Autodesk Inventor part; units mm, degrees
ref_plane "YZ Plane" through (0, 0, 0) normal (1, 0, 0) x (0, 1, 0)
ref_plane "XZ Plane" through (0, 0, 0) normal (0, 1, 0) x (-1, 0, 0)
ref_plane "XY Plane" through (0, 0, 0) normal (0, 0, 1) x (1, 0, 0)
ref_plane "Work Plane1" through (0, 0, 0) normal (0, 0, 1) x (1, 0, 0)
sketch "Sketch1" plane through (0, 0, 0) normal (0, 0, 1) x (1, 0, 0)
  circle A0 centre (11.5562, -18) radius 2 construction
  line L0 (-53.1938, -16) -> (-53.1938, -30) construction
  arc A1 (-56.1938, -30) -> (-53.1938, -30) centre (-54.6938, -30) ccw construction
  line L1 (-56.1938, -30) -> (-56.1938, -16) construction
  arc A2 (-53.1938, -16) -> (-56.1938, -16) centre (-54.6938, -16) ccw construction
  line L2 (7.0562, -16) -> (7.0562, -30) construction
  arc A3 (4.0562, -30) -> (7.0562, -30) centre (5.5562, -30) ccw construction
  line L3 (4.0562, -30) -> (4.0562, -16) construction
  arc A4 (7.0562, -16) -> (4.0562, -16) centre (5.5562, -16) ccw construction
  line L4 (-13.1938, -16) -> (-13.1938, -30) construction
  arc A5 (-16.1938, -30) -> (-13.1938, -30) centre (-14.6938, -30) ccw construction
  line L5 (-16.1938, -30) -> (-16.1938, -16) construction
  arc A6 (-13.1938, -16) -> (-16.1938, -16) centre (-14.6938, -16) ccw construction
  arc A7 (19.0562, -16) -> (16.0562, -16) centre (17.5562, -16) ccw construction
  line L6 (19.0562, -16) -> (19.0562, -30) construction
  arc A8 (16.0562, -30) -> (19.0562, -30) centre (17.5562, -30) ccw construction
  line L7 (16.0562, -30) -> (16.0562, -16) construction
  line L8 (22.8064, -40) -> (22.8064, 45) construction
  line L9 (22.8064, 45) -> (-120, 45) construction
  line L10 (-120, 27.5563) -> (-120, 45) construction
  line L11 (-120, 27.5563) -> (-95.2035, 27.5563) construction
  arc A9 (-85.0841, 27.5563) -> (-95.2035, 27.5563) centre (-90.1438, 25.4) ccw construction
  line L12 (-85.0841, 27.5563) -> (17.8062, 27.5563) construction
  line L13 (17.8062, 27.5563) -> (17.8062, -11) construction
  line L14 (17.8062, -11) -> (-120, -11) construction
  line L15 (-120, -40) -> (-120, -11) construction
  line L16 (22.8064, -40) -> (-120, -40) construction
  circle A10 centre (-111.1938, -18) radius 2 construction
  circle A11 centre (-98.1938, -18) radius 2 construction
  circle A12 centre (-61.1938, -18) radius 2 construction
  circle A13 centre (-48.1938, -18) radius 2 construction
  circle A14 centre (-21.1938, -18) radius 2 construction
  circle A15 centre (-8.1938, -18) radius 2 construction
  circle A16 centre (-21.1938, 33.6563) radius 2 construction
  circle A17 centre (-8.1938, 33.6563) radius 2 construction
  circle A18 centre (-61.1938, 33.6563) radius 2 construction
  circle A19 centre (-48.1938, 33.6563) radius 2 construction
  circle A20 centre (-111.1938, 33.6563) radius 2 construction
  circle A21 centre (-98.1938, 33.6563) radius 2 construction
  circle A22 centre (-90.1438, -25.4) radius 5.5 construction
  circle A23 centre (7.8062, 0) radius 3.75 construction
  circle A24 centre (-24.6938, 0) radius 3.75 construction
  line L17 (22.8064, -35.5) -> (-39.6938, -35.5)
  line L18 (-39.6938, -35.5) -> (-39.6938, 0)
  line L19 (-39.6938, 0) -> (-28.5438, 0)
  line L20 (22.8064, 0) -> (22.8064, -35.5)
  line L21 (-34.6938, -11) -> (-34.6938, 11) construction
  arc A25 (3.9562, 0) -> (11.6562, 0) centre (7.8062, 0) ccw
  line L22 (11.6562, 0) -> (22.8064, 0)
  arc A26 (-28.5438, 0) -> (-20.8438, 0) centre (-24.6938, 0) ccw
  line L23 (-20.8438, 0) -> (3.9562, 0)
  point P0 (0, 0)
  point P1 (17.5562, -31.5)
  dimension "d0" = 5
  dimension "d1" = 0
  dimension "d2" = 0.1
  dimension "d3" = 0.1
  dimension "d4" = 4
extrude "Main Body" add sketch "Sketch1" along normal blind 5
sketch "Sketch2" plane through (0, 0, 0) normal (0, 0, -1) x (-1, 0, 0)
  line L0 (16.1938, -30) -> (16.1938, -16) construction
  arc A0 (13.1938, -30) -> (16.1938, -30) centre (14.6938, -30) ccw construction
  line L1 (13.1938, -16) -> (13.1938, -30) construction
  arc A1 (16.1938, -16) -> (13.1938, -16) centre (14.6938, -16) ccw construction
  line L2 (16.1938, -30) -> (16.1938, -16) construction
  line L3 (-4.0562, -30) -> (-4.0562, -16) construction
  arc A2 (-7.0562, -30) -> (-4.0562, -30) centre (-5.5562, -30) ccw construction
  line L4 (-7.0562, -16) -> (-7.0562, -30) construction
  arc A3 (-4.0562, -16) -> (-7.0562, -16) centre (-5.5562, -16) ccw construction
  line L5 (-5.5562, -16) -> (-5.5562, -30) construction
  line L6 (14.6938, -16) -> (14.6938, -30) construction
  line L7 (-5.5562, -17) -> (-5.5562, -29) construction
  line L8 (-7.0062, -17) -> (-7.0062, -29)
  line L9 (-4.1062, -29) -> (-4.1062, -17)
  arc A4 (-4.1062, -17) -> (-7.0062, -17) centre (-5.5562, -17) ccw
  arc A5 (-7.0062, -29) -> (-4.1062, -29) centre (-5.5562, -29) ccw
  line L10 (14.6938, -17) -> (14.6938, -29) construction
  line L11 (13.2438, -17) -> (13.2438, -29)
  line L12 (16.1438, -29) -> (16.1438, -17)
  arc A6 (16.1438, -17) -> (13.2438, -17) centre (14.6938, -17) ccw
  arc A7 (13.2438, -29) -> (16.1438, -29) centre (14.6938, -29) ccw
  line L13 (-5.5562, -17) -> (14.6938, -17) construction
  line L14 (-5.5562, -29) -> (14.6938, -29) construction
  point P0 (0, 0)
  point P1 (-5.5562, -23)
  point P2 (14.6938, -23)
  dimension "d9" = 0.05
  dimension "d10" = 0.05
  dimension "d11" = 1
  dimension "d12" = 1
extrude "Alignment Tabs" add sketch "Sketch2" along normal blind 1.8
sketch "Sketch3" plane through (0, 0, 5) normal (0, 0, 1) x (1, 0, 0)
  circle A0 centre (-8.1938, -18) radius 2 construction
  line L0 (-8.1938, -31.3066) -> (-8.1938, -7.4741) construction
  line L1 (-8.1938, -16.5) -> (-8.1938, -19.5) construction
  line L2 (-6.4438, -16.5) -> (-6.4438, -19.5)
  line L3 (-9.9438, -19.5) -> (-9.9438, -16.5)
  arc A1 (-6.4438, -16.5) -> (-9.9438, -16.5) centre (-8.1938, -16.5) ccw
  arc A2 (-9.9438, -19.5) -> (-6.4438, -19.5) centre (-8.1938, -19.5) ccw
  point P0 (0, 0)
  dimension "d14" = 3.5
  dimension "d15" = 3
extrude "Slot for Screw M3" cut sketch "Sketch3" against normal through all
equation "\"d3\" = d2"
equation "\"d10\" = d9"
equation "\"d12\" = d11"
properties part number "Cuvette Aligner 50mm"
Build history of the part. All positions in model axes, mm. A direction names the side the tool comes from. Coordinates: 2 decimals unless noted, no trailing zeros. Order: outer loops, then holes, each group sorted by start corner. A loop starts at its lowest first (then second) coordinate and runs counter-clockwise, first axis right, second up. Notation, with made-up numbers: (59, 73.25) -> (64, 73.25) arc R24 ccw to (64, 109.25) -> close; hole circle Ø1 at (-11.75, 24). An arc over 180 degrees is marked (long way). Answer in a Markdown table with one row per item. Add a question column.
Q1. Band-saw the part on D-D, the plane x = -15. List the corners of the cut face in (y, z), then the cut area to 3 significant figures.
Q2. Drop flat-ended pins along their axis: pin 1 (10 mm diameter, centred on x = -3, y = -16, fed in from -Z); pin 2 (1.4 mm diameter, centred on y = -24, z = -1.5, fed in from +X); pin 3 (0.9 mm diameter, centred on y = -20.5, z = -1, fed in from -X); pin 4 (18 mm diameter, centred on x = -1.5, y = -19.5, fed in from -Z). Give the stop position or say it passes through.
Q3. Band-saw the part on B-B, the plane z = 2.25. List the corners of the cut face in (x, y), then the cut area to 3 significant figures.
Q4. Mould opens along Y. For faces 6 (the face through (22.806, -18, 2)), 7 (the face through (-14.73, -30.45, -0.89)), 8 (the face through (-9.944, -18, 3)) say: +Y half, -Y half, draft (parallel to the pull), parting line (faces both ways), or undercut.
Q5. Which spindle directions (+Z, -Z, +X, -X, +Y, -Y) get a long thin tool onto all of the face, cutting with end or side? Do faces 1 (the face through (4.106, -23, -1)), 2 (the face through (5.52, -30.45, -0.89)), 3 (the face through (5.59, -15.55, -0.89)), 4 (the face through (-8.16, -14.75, 2.54)), 5 (the face through (-16.144, -23, -1)). Say none if no direction does.
Q6. Band-saw the part on A-A, the plane y = -18. List the corners of the cut face in (x, z).
Q7. Band-saw the part on C-C, the plane y = -25.5. List the corners of the cut face in (x, z), then the cut area to 3 significant figures.
Q8. Wall check: line 1 along X through (y, z) = (-19.5, 0.75); line 2 along X through (y, z) = (-25, -1.25); line 3 along Z through (x, y) = (4.5, -10). Give the ranges that are in metal, low to high. Write a range as [from, to].
Answers follow:
| question | item | result |
|---|---|---|
| 1 | outline | (-35.5, 0) -> (-30.42, 0) -> (-30.42, -1.8) -> (-15.58, -1.8) -> (-15.58, 0) -> (0, 0) -> (0, 5) -> (-35.5, 5) -> close |
| 1 | area | 204 mm^2 |
| 2 | pin 1 | z = 0 |
| 2 | pin 2 | x = 7.01 |
| 2 | pin 3 | x = -16.14 |
| 2 | pin 4 | z = -1.8 |
| 3 | outline | (-39.69, -35.5) -> (22.81, -35.5) -> (22.81, 0) -> (11.66, 0) arc R3.85 cw to (3.96, 0) -> (-20.84, 0) arc R3.85 cw to (-28.54, 0) -> (-39.69, 0) -> close; hole (-9.94, -19.5) arc R1.75 ccw to (-6.44, -19.5) -> (-6.44, -16.5) arc R1.75 ccw to (-9.94, -16.5) -> close |
| 3 | area | 2,150 mm^2 |
| 4 | face 6 | draft |
| 4 | face 7 | -Y half |
| 4 | face 8 | undercut |
| 5 | face 1 | -Z, +Y, -Y |
| 5 | face 2 | -Z, -Y |
| 5 | face 3 | -Z, +Y |
| 5 | face 4 | +Z, -Z |
| 5 | face 5 | -Z, -X, +Y, -Y |
| 6 | outline | (-39.69, 0) -> (-16.14, 0) -> (-16.14, -1.8) -> (-13.24, -1.8) -> (-13.24, 0) -> (-9.94, 0) -> (-9.94, 5) -> (-39.69, 5) -> close; (-6.44, 0) -> (4.11, 0) -> (4.11, -1.8) -> (7.01, -1.8) -> (7.01, 0) -> (22.81, 0) -> (22.81, 5) -> (-6.44, 5) -> close |
| 7 | outline | (-39.69, 0) -> (-16.14, 0) -> (-16.14, -1.8) -> (-13.24, -1.8) -> (-13.24, 0) -> (4.11, 0) -> (4.11, -1.8) -> (7.01, -1.8) -> (7.01, 0) -> (22.81, 0) -> (22.81, 5) -> (-39.69, 5) -> close |
| 7 | area | 323 mm^2 |
| 8 | line 1 | [-39.69, -9.94], [-6.44, 22.81] |
| 8 | line 2 | [-16.14, -13.24], [4.11, 7.01] |
| 8 | line 3 | [0, 5] |
